from build123d import *

# Parameters (mm, degrees)
F0_R     = 1.7
F0_R_2   = 0.75
F1_DEPTH = 6
F2_R     = 2.330452
F2_R_2   = 1.7
F2_R_3   = 2.349172
F3_DEPTH = 3
F4_R     = 2.25
F4_R_2   = 0.75
F5_DEPTH = 2.6


with BuildPart() as f1:
    # F0 (on Top) → F1 (new body)
    with BuildSketch(Plane.XY):
        Polygon((12.663894, 0), (12.663894, 3.477627), (-12.663894, 3.477627), (-12.663894, -2.954399), (12.663894, -2.954399), align=None)
        with Locations((-9.565, 0)):
            Circle(F0_R, mode=Mode.SUBTRACT)
        with Locations((-3.615, 0)):
            Circle(F0_R_2, mode=Mode.SUBTRACT)
        with Locations((3.615, 0)):
            Circle(F0_R_2, mode=Mode.SUBTRACT)
        with Locations((9.565, 0)):
            Circle(F0_R, mode=Mode.SUBTRACT)
    extrude(amount=F1_DEPTH)

    # F2 (on face) → F3 (cut)
    with BuildSketch(Plane.XY.offset(6)):
        with Locations((-9.565, 0)):
            Circle(F2_R)
        with Locations((-9.565, 0)):
            Circle(F2_R_2, mode=Mode.SUBTRACT)
        with Locations((9.565, 0)):
            Circle(F2_R_3)
        with Locations((9.565, 0)):
            Circle(F2_R_2, mode=Mode.SUBTRACT)
    extrude(amount=-F3_DEPTH, mode=Mode.SUBTRACT)

    # F4 (on face) → F5 (cut)
    with BuildSketch(Plane(origin=(0, 0, 0), x_dir=(1, 0, 0), z_dir=(0, 0, -1))):
        with Locations((-3.615, 0)):
            Circle(F4_R)
        with Locations((-3.615, 0)):
            Circle(F4_R_2, mode=Mode.SUBTRACT)
        with Locations((3.615, 0)):
            Circle(F4_R)
        with Locations((3.615, 0)):
            Circle(F4_R_2, mode=Mode.SUBTRACT)
    extrude(amount=-F5_DEPTH, mode=Mode.SUBTRACT)


solid = f1.part
Can you work these out from the model? Positions are in its coordinate system, mm. A direction names the side the tool comes from. Give positions to 0.01 mm unless a question says otherwise; leave off trailing zeros. Loops run counter-clockwise (first coordinate to the right, second up) from the corner with the lowest first, then second, coordinate; pieces in that order, holes last. Notation, with made-up numbers: (37, 27) -> (63, 27) arc R31 ccw to (63, 64) -> close; hole circle Ø7 at (33.5, -32). An arc over 180 degrees is marked (long way). Use one line per item in the form item = value.
1) If we section it at A-A (z = 3.8): Please give me the cut outline in (x, y) (3 decimals).
Answers:
outline = (-12.664, -2.954) -> (12.664, -2.954) -> (12.664, 3.478) -> (-12.664, 3.478) -> close; hole circle Ø4.661 at (-9.565, 0); hole circle Ø1.5 at (-3.615, 0); hole circle Ø1.5 at (3.615, 0); hole circle Ø4.698 at (9.565, 0)
2) We'd pull the mould along Y, two halves only. Please class faces 1 (the face through (7.867, 0.075, 1.479)), 2 (the face through (0, -2.954, 3)), 3 (the face through (0, 0, 6)): released by +Y, released by -Y, zero draft, split by the parting line, or undercut.
Answers:
face_1 = undercut
face_2 = released by -Y
face_3 = zero draft
3) If we section it at D-D (y = 0): Count the separate pieces of the cut face and the enclosed holes in it, plus the area to 3 significant figures.
Answers:
separate_pieces = 5
enclosed_holes = 0
area = 69.9 mm²
4) For faces 4 (the face through (3, -1, 2.6)), 5 (the face through (4.308, -0.287, 4.276)), 6 (the face through (7.218, 0.103, 4.521)), which set-ups out of +Z, -Z, +X, -X, +Y, -Y let a thin tool reach every point of the face, with its end or its side?
Answers:
face_4 = -Z
face_5 = +Z, -Z
face_6 = +Z
5) I need wall thicknesses on line 1 along X through (y, z) = (-0.5, 0.9); line 2 along X through (y, z) = (1.25, 0.95); line 3 along Z through (x, y) = (7.75, 1). Which ranges of each line are inside material? Lowest first, please.
Answers:
line_1 = -12.66 to -11.19, -7.94 to -5.81, -1.42 to 1.42, 5.81 to 7.94, 11.19 to 12.66
line_2 = -12.66 to -10.72, -8.41 to -5.49, -1.74 to 1.74, 5.49 to 8.41, 10.72 to 12.66
line_3 = 0 to 3
6) If we section it at C-C (y = -2): Please give me the cut outline in (x, z).
Answers:
outline = (-12.66, 0) -> (-4.65, 0) -> (-4.65, 2.6) -> (-2.58, 2.6) -> (-2.58, 0) -> (2.58, 0) -> (2.58, 2.6) -> (4.65, 2.6) -> (4.65, 0) -> (12.66, 0) -> (12.66, 6) -> (10.8, 6) -> (10.8, 3) -> (8.33, 3) -> (8.33, 6) -> (-8.37, 6) -> (-8.37, 3) -> (-10.76, 3) -> (-10.76, 6) -> (-12.66, 6) -> close
7) Will this pin go through, and if not, where does the flat tip stop? pin 1 (1.3 mm diameter, centred on x = -3.5, y = -0.5, fed in from -Z).
Answers:
pin_1 = 2.6
8) If we section it at B-B (x = 3.5): Please give me the cut outline in (y, z), plus the area to 3 significant figures.
Answers:
outline = (-2.95, 0) -> (-2.25, 0) -> (-2.25, 2.6) -> (-0.74, 2.6) -> (-0.74, 6) -> (-2.95, 6) -> close; (0.74, 2.6) -> (2.25, 2.6) -> (2.25, 0) -> (3.48, 0) -> (3.48, 6) -> (0.74, 6) -> close
area = 21.9 mm²
